Geometry: see drawing. Coordinates: mm, zero at the bounding-box minimum. Coordinates: 2 decimals unless noted, no trailing zeros. Loops run counter-clockwise (first coordinate to the right, second up) from the corner with the lowest first, then second, coordinate; pieces in that order, holes last. Notation, with made-up numbers: M 30.5,46.25 L 46.5,46.25 A18 cw 46.5,53.25 Z; hole C 53.25,-38 d2. An arc over 180 degrees is marked long. One line per question, with ' | ' between items. Start each with the question number.
1. Ray query, probe 1 along X at (y, z) = (279.4, 5.75); probe 2 along Y at (x, z) = (50.8, 5.75); probe 3 along X at (y, z) = (279.4, 11.5). Return the intervals inside material, ascending.
2. Section query A-A, the plane y = 279.4. Output: boundary loops of the cut face in (x, z).
3. Section query C-C, the plane x = 50.8. Output: boundary loops of the cut face in (y, z), and give its area (3 significant figures).
4. Section query B-B, the plane z = 9.5. Output: boundary loops of the cut face in (x, y), and give its area (3 significant figures).
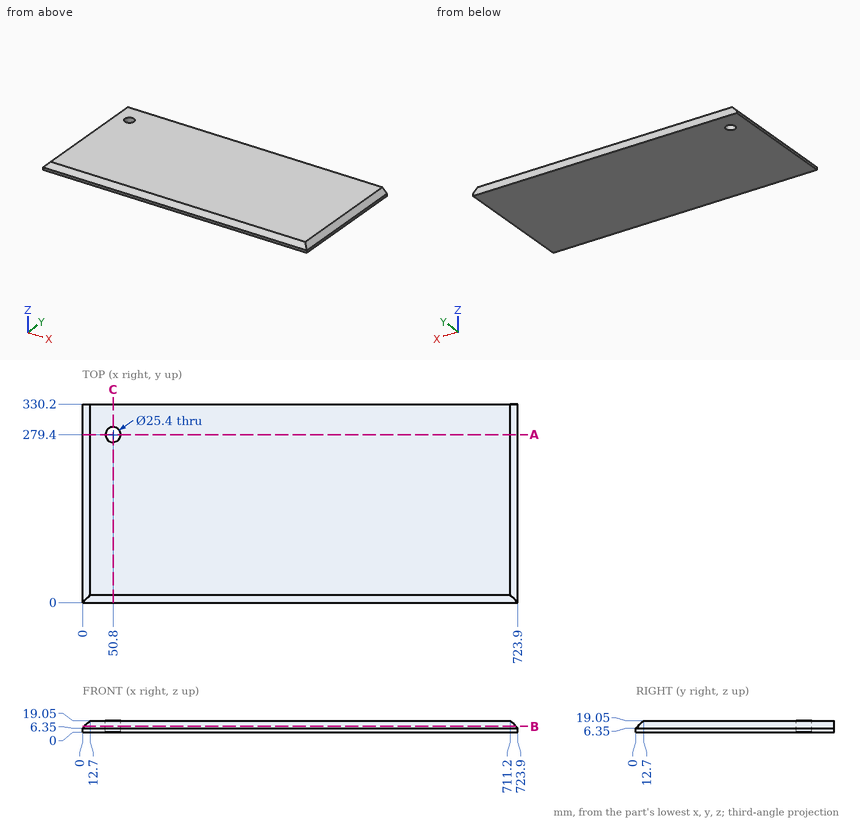
Taken from the geometry:
1) probe 1: 0 to 38.1, 63.5 to 723.9 | probe 2: 0 to 266.7, 292.1 to 330.2 | probe 3: 5.15 to 38.1, 63.5 to 718.75
2) outline: M 0,0 L 38.1,0 L 38.1,19.05 L 12.7,19.05 L 0,6.35 Z; M 63.5,0 L 723.9,0 L 723.9,6.35 L 711.2,19.05 L 63.5,19.05 Z
3) outline: M 0,0 L 266.7,0 L 266.7,19.05 L 12.7,19.05 L 0,6.35 Z; M 292.1,0 L 330.2,0 L 330.2,19.05 L 292.1,19.05 Z | area: 5,730 mm^2
4) outline: M 3.15,3.15 L 720.75,3.15 L 720.75,330.2 L 3.15,330.2 Z; hole C 50.8,279.4 d25.4 | area: 234,000 mm^2
